from build123d import *

# Parameters (mm, degrees)
BOSS_EXTRUDE1_DEPTH = 10.16
SKETCH2_W           = 38.1
SKETCH2_H           = 9.5
CUT_EXTRUDE1_DEPTH  = 2540


with BuildPart() as part:
    # Sketch1 → Boss-Extrude1 (new body)
    with BuildSketch(Plane.XY):
        Polygon((-123.444, 2072.64), (-205.715298803, 2072.64), (-205.715298803, 2052.32), (-215.881789204, 2052.32), (-215.881789204, 1963.42), (-205.715298803, 1963.42), (-205.715298803, 1874.52), (-215.881789204, 1874.52), (-215.881789204, 1785.62), (-205.715298803, 1785.62), (-205.715298803, 1696.72), (-215.875298803, 1696.72), (-215.875298803, 1607.82), (-205.715298803, 1607.82), (-205.715298803, 1518.92), (-215.881789204, 1518.92), (-215.881789204, 1488.440000035), (-358.121789204, 1488.440000035), (-358.121789204, 20.32), (-303.52, 20.32), (-303.52, 0), (-252, 0), (-252, 20.32), (-55.8292, 20.32), (-55.8292, 0), (55.8292, 0), (55.8292, 20.32), (252, 20.32), (252, 0), (303.52, 0), (303.52, 20.32), (358.121789204, 20.32), (358.121789204, 1488.440000035), (215.881789204, 1488.440000035), (215.881789204, 1518.92), (205.715298803, 1518.92), (205.715298803, 1607.82), (215.875298803, 1607.82), (215.875298803, 1696.72), (205.715298803, 1696.72), (205.715298803, 1785.62), (215.881789204, 1785.62), (215.881789204, 1874.52), (205.715298803, 1874.52), (205.715298803, 1963.42), (215.881789204, 1963.42), (215.881789204, 2052.32), (205.715298803, 2052.32), (205.715298803, 2072.64), (123.444, 2072.64), (123.444, 2052.32), (41.135649402, 2052.32), (41.135649402, 2072.64), (-41.135649402, 2072.64), (-41.135649402, 2052.32), (-123.444, 2052.32), align=None)
        Polygon((215.881789204, 1463.040000035), (222.040744894, 1374.366931824), (211.92306481, 1373.664189215), (205.715298803, 1463.040000035), align=None, mode=Mode.SUBTRACT)
        Polygon((-205.715298803, 1463.040000035), (-211.92306481, 1373.664189215), (-222.040744894, 1374.366931824), (-215.881789204, 1463.040000035), align=None, mode=Mode.SUBTRACT)
        Polygon((227.836927701, 1290.916856945), (234.358656272, 1197.020795404), (224.240976188, 1196.318052795), (217.719247617, 1290.214114336), align=None, mode=Mode.SUBTRACT)
        Polygon((-308.266124544, 132.94397688), (-301.755453134, 226.680843836), (-291.63777305, 225.978101227), (-298.14844446, 132.241234271), align=None, mode=Mode.SUBTRACT)
        Polygon((-289.435698895, 404.053512688), (-279.318018811, 403.350770078), (-285.830533081, 309.587370692), (-295.948213166, 310.290113301), align=None, mode=Mode.SUBTRACT)
        Polygon((-283.630301787, 487.636249721), (-277.115944656, 581.426181539), (-266.998264572, 580.72343893), (-273.512621703, 486.933507112), align=None, mode=Mode.SUBTRACT)
        Polygon((-264.796190418, 758.798850391), (-254.678510334, 758.096107781), (-261.194710324, 664.279643533), (-271.312390408, 664.982386142), align=None, mode=Mode.SUBTRACT)
        Polygon((-252.476436179, 936.171519242), (-242.358756095, 935.468776633), (-248.876798945, 841.625779953), (-258.99447903, 842.328522563), align=None, mode=Mode.SUBTRACT)
        Polygon((301.755453134, 226.680843836), (308.266124544, 132.94397688), (298.14844446, 132.241234271), (291.63777305, 225.978101227), align=None, mode=Mode.SUBTRACT)
        Polygon((279.318018811, 403.350770078), (289.435698895, 404.053512688), (295.948213166, 310.290113301), (285.830533081, 309.587370692), align=None, mode=Mode.SUBTRACT)
        Polygon((254.678510334, 758.096107781), (264.796190418, 758.798850391), (271.312390408, 664.982386142), (261.194710324, 664.279643533), align=None, mode=Mode.SUBTRACT)
        Polygon((277.115944656, 581.426181539), (283.630301787, 487.636249721), (273.512621703, 486.933507112), (266.998264572, 580.72343893), align=None, mode=Mode.SUBTRACT)
        Polygon((242.358756095, 935.468776633), (252.476436179, 936.171519242), (258.99447903, 842.328522563), (248.876798945, 841.625779953), align=None, mode=Mode.SUBTRACT)
        Polygon((-240.15668194, 1113.544188093), (-230.039001856, 1112.841445484), (-236.558887567, 1018.971916374), (-246.676567651, 1019.674658983), align=None, mode=Mode.SUBTRACT)
        Polygon((-227.836927701, 1290.916856945), (-217.719247617, 1290.214114336), (-224.240976188, 1196.318052795), (-234.358656272, 1197.020795404), align=None, mode=Mode.SUBTRACT)
        Polygon((230.039001856, 1112.841445484), (240.15668194, 1113.544188093), (246.676567651, 1019.674658983), (236.558887567, 1018.971916374), align=None, mode=Mode.SUBTRACT)
    extrude(amount=BOSS_EXTRUDE1_DEPTH)

    # Sketch2 → Cut-Extrude1 (cut)
    with BuildSketch(Plane(origin=(0, 0, 0), x_dir=(1, 0, 0), z_dir=(0, 1, 0))):
        with Locations((339.071789204, -4.75)):
            Rectangle(SKETCH2_W, SKETCH2_H)
        with Locations((-339.071789204, -4.75)):
            Rectangle(SKETCH2_W, SKETCH2_H)
    extrude(amount=CUT_EXTRUDE1_DEPTH, mode=Mode.SUBTRACT)


solid = part.part
Here's how the part is built. I have some questions about the finished solid (model axes, mm). A direction names the side the tool comes from. Give positions to 0.01 mm unless a question says otherwise; leave off trailing zeros. Order: outer loops, then holes, each group sorted by start corner. A loop starts at its lowest first (then second) coordinate and runs counter-clockwise, first axis right, second up. Notation, with made-up numbers: M 42.25,44 L 74.25,44 A16 cw 74.25,65 Z; hole C -37,22 d5. An arc over 180 degrees is marked long. Answer as a JSON object with one key per item and string values. Group by question number.
1) Suppose I cut it at D-D, the plane z = 5. Count the separate pieces of the cut face and the enclosed holes in it, plus the area to 3 significant figures.
2) Suppose I cut it at C-C, the plane x = -95.5. Write out the boundary of the cut face in (y, z).
3) Please list where these lines run through material, in increasing order: L1, parallel to Y at x = -277, z = 3.75; L2, parallel to Y at x = 301.5, z = 3; L3, parallel to X at y = 1950, z = 9. Write a range as [from, to].
4) Suppose I cut it at A-A, the plane y = 1173.5. Write out the boundary of the cut face in (x, z).
5) Suppose I cut it at B-B, the plane y = 169.5. Write out the boundary of the cut face in (x, z), plus the area to 3 significant figures.
6) On a 3-axis mill with a long thin cutter (end or side, diameter ignored), from which of +Z, -Z, +X, -X, +Y, -Y can I reach the whole of each face in a straight line? I mean faces 1 (the flat face through (339, 744, 9.5)), 2 (the flat face through (-5, 821, 10.16)), 3 (the flat face through (-339, 744, 9.5)). Say none if no direction works.
7) I'm going to push flat-ended pins straight in: pin 1 Ø4 at (x, z) = (-197, 1.5) entering from -Y; pin 2 Ø4 at (x, z) = (101.5, 3) entering from +Y; pin 3 Ø1.5 at (y, z) = (1031.5, 1.5) entering from -X. Where does each tip first touch, or does it pass through?
Results found:
{
 "1": {"separate pieces": "1", "enclosed holes": "16", "area": "1,170,000 mm²"},
 "2": {"outline": "M 20.32,0 L 2052.32,0 L 2052.32,10.16 L 20.32,10.16 Z"},
 "3": {"L1": "[0, 487.18], [581.42, 1488.44]", "L2": "[0, 132.47], [226.66, 1488.44]", "L3": "[-205.72, 205.72]"},
 "4": {"outline": "M -358.12,9.5 L -320.02,9.5 L -320.02,0 L 320.02,0 L 320.02,9.5 L 358.12,9.5 L 358.12,10.16 L -358.12,10.16 Z"},
 "5": {"outline": "M -358.12,9.5 L -320.02,9.5 L -320.02,0 L -305.73,0 L -305.73,10.16 L -358.12,10.16 Z; M -295.56,0 L 295.56,0 L 295.56,10.16 L -295.56,10.16 Z; M 305.73,0 L 320.02,0 L 320.02,9.5 L 358.12,9.5 L 358.12,10.16 L 305.73,10.16 Z", "area": "6,350 mm²"},
 "6": {"face 1": "-Z, +X, +Y, -Y", "face 2": "+Z, +X, -X, +Y, -Y", "face 3": "-Z, -X, +Y, -Y"},
 "7": {"pin 1": "y = 20.32", "pin 2": "y = 2052.32", "pin 3": "x = -320.02"}
}
